```python
from build123d import *

# Parameters (mm, degrees)
F0_W      = 76.2
F0_H      = 44.45
F1_DEPTH  = 25.4
F2_W      = 25.4
F2_H      = 31.75
F3_DEPTH  = 25.4
F5_DEPTH  = 25.4
F6_R      = 6.4097616639
F7_DEPTH  = 25.4
F9_DEPTH  = 25.4
F11_DEPTH = 25.4
F12_R     = 6.9616762065
F12_R_2   = 6.701591824
F13_DEPTH = 25.4


with BuildPart() as f1:
    # F0 (on Front) → F1 (new body)
    with BuildSketch(Plane.XZ):
        with Locations((38.1, 22.225)):
            Rectangle(F0_W, F0_H)
    extrude(amount=F1_DEPTH)

    # F2 (on face) → F3 (cut)
    with BuildSketch(Plane.XZ.offset(25.4)):
        with Locations((12.7, 28.575)):
            Rectangle(F2_W, F2_H)
        with Locations((63.5, 28.575)):
            Rectangle(F2_W, F2_H)
    extrude(amount=-F3_DEPTH, mode=Mode.SUBTRACT)

    # F4 (on face) → F5 (cut)
    with BuildSketch(Plane.YZ.offset(50.8)):
        with BuildLine():
            ThreePointArc((-25.4, 37.343819084), (-21.8851025395, 42.054991557), (-16.517273855, 44.45))
            Line((-16.517273855, 44.45), (-25.4, 44.45))
            Line((-25.4, 44.45), (-25.4, 37.343819084))
        make_face()
        with BuildLine():
            Line((0, 44.45), (-12.7, 44.45))
            ThreePointArc((-12.7, 44.45), (-4.2917980427, 40.8099765707), (0, 32.7150336876))
            Line((0, 32.7150336876), (0, 44.45))
        make_face()
    extrude(amount=-F5_DEPTH, mode=Mode.SUBTRACT)

    # F6 (on face) → F7 (cut)
    with BuildSketch(Plane.YZ.offset(50.8)):
        with Locations((-13.6843539452, 30.6450168438)):
            Circle(F6_R)
    extrude(amount=-F7_DEPTH, mode=Mode.SUBTRACT)

    # F8 (on face) → F9 (cut)
    with BuildSketch(Plane.XY.offset(12.7)):
        with BuildLine():
            Line((0, 0), (0, -9.0078908736))
            ThreePointArc((0, -9.0078908736), (2.3832082238, -3.5743776274), (7.1188784204, 0))
            Line((7.1188784204, 0), (0, 0))
        make_face()
        with BuildLine():
            ThreePointArc((7.1188784204, -25.4), (2.2814327848, -21.4359106329), (0, -15.612685647))
            Line((0, -15.612685647), (0, -25.4))
            Line((0, -25.4), (7.1188784204, -25.4))
        make_face()
    extrude(amount=-F9_DEPTH, mode=Mode.SUBTRACT)

    # F10 (on face) → F11 (cut)
    with BuildSketch(Plane.XY.offset(12.7)):
        with BuildLine():
            ThreePointArc((67.3354417086, 0), (73.7069873412, -4.7726544119), (76.2, -12.3330586186))
            Line((76.2, -12.3330586186), (76.2, 0))
            Line((76.2, 0), (67.3354417086, 0))
        make_face()
        with BuildLine():
            ThreePointArc((76.2, -14.8152652197), (73.4320785831, -21.5015075072), (67.3354417086, -25.4))
            Line((67.3354417086, -25.4), (76.2, -25.4))
            Line((76.2, -25.4), (76.2, -14.8152652197))
        make_face()
    extrude(amount=-F11_DEPTH, mode=Mode.SUBTRACT)

    # F12 (on face) → F13 (cut)
    with BuildSketch(Plane.XY.offset(12.7)):
        with Locations((62.8318414092, -12.3102882603)):
            Circle(F12_R)
        with Locations((15.475823544, -12.3102882603)):
            Circle(F12_R_2)
    extrude(amount=-F13_DEPTH, mode=Mode.SUBTRACT)


solid = f1.part
```
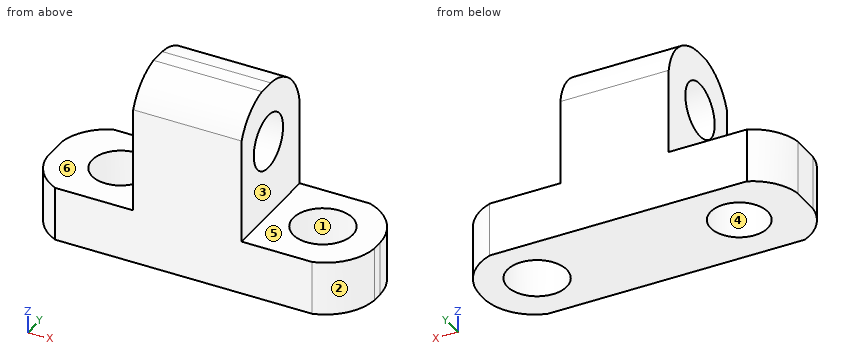
Input: part model. Units: mm. Frame: model coordinates. Face numbers are marked on the shaded views. A direction names the side the tool comes from. Round coordinates to 2 decimals unless told otherwise and drop trailing zeros. Order: outer loops, then holes, each group sorted by start corner. A loop starts at its lowest first (then second) coordinate and runs counter-clockwise, first axis right, second up. Notation, with made-up numbers: (61.25, 80) - (65.25, 80) arc R27 ccw to (65.25, 112) - close; hole circle Ø3 at (-39.75, 69). An arc over 180 degrees is marked (long way). Answer in a Markdown table with one row per item.
Item 1: Section query D-D (x = 42.5). Return the cut outline in (y, z).
Model answer:
| item | result |
|---|---|
| outline | (-25.4, 0) - (0, 0) - (0, 32.72) arc R13.84 ccw to (-12.7, 44.45) - (-16.52, 44.45) arc R11.65 ccw to (-25.4, 37.34) - close; hole circle Ø12.82 at (-13.68, 30.65) |
Item 2: Reachability of the marked faces 4, 5 and 6 from +Z, -Z, +X, -X, +Y, -Y: full face, straight path, thin tool, end or side. Return the list, or none.
Model answer:
| item | result |
|---|---|
| face 4 | +Z, -Z |
| face 5 | +Z, +X, +Y, -Y |
| face 6 | +Z, -X, +Y, -Y |
Item 3: Pin query (flat end, axial travel): pin 1 (10.5 mm diameter, centred on y = -13.68, z = 30.65, fed in from +X); pin 2 (1.5 mm diameter, centred on y = -17, z = 15.5, fed in from -X); pin 3 (8 mm diameter, centred on y = -17, z = 22.5, fed in from +X); pin 4 (7.5 mm diameter, centred on x = 15.5, y = -6.5, fed in from +Z). Return the tip coordinate at first contact, or that it passes through.
Model answer:
| item | result |
|---|---|
| pin 1 | passes through |
| pin 2 | stops at x = 25.4 |
| pin 3 | stops at x = 50.8 |
| pin 4 | stops at z = 12.7 |
Item 4: Section query C-C (z = 7.5). Return the cut outline in (x, y).
Model answer:
| item | result |
|---|---|
| outline | (0, -15.61) arc R12.38 ccw to (7.12, -25.4) - (67.34, -25.4) arc R12.06 ccw to (76.2, -14.82) - (76.2, -12.33) arc R13.27 ccw to (67.34, 0) - (7.12, 0) arc R11.74 ccw to (0, -9.01) - close; hole circle Ø13.4 at (15.48, -12.31); hole circle Ø13.92 at (62.83, -12.31) |
Item 5: Line query: line 1 (X direction, y = -12, z = 5); line 2 (X direction, y = -13, z = 38.5); line 3 (Z direction, x = 55, y = -10.5). Output: solid intervals per line, ascending.
Model answer:
| item | result |
|---|---|
| line 1 | x = 0 to 8.78, 22.17 to 55.88, 69.79 to 76.19 |
| line 2 | x = 25.4 to 50.8 |
| line 3 | z = 0 to 12.7 |
Item 6: Section query A-A (x = 59). Return the cut outline in (y, z).
Model answer:
| item | result |
|---|---|
| outline | (-25.4, 0) - (-18.12, 0) - (-18.12, 12.7) - (-25.4, 12.7) - close; (-6.5, 0) - (0, 0) - (0, 12.7) - (-6.5, 12.7) - close |
Item 7: Mould query, pull axis Y, two halves, no side actions, for the marked faces 1, 2 and 3. Classes: released by +Y, released by -Y, zero draft, split by the parting line, or undercut.
Model answer:
| item | result |
|---|---|
| face 1 | undercut |
| face 2 | released by -Y |
| face 3 | zero draft |
Item 8: Section query B-B (z = 25). Return the cut outline in (x, y), then the cut area to 3 significant figures.
Model answer:
| item | result |
|---|---|
| outline | (25.4, -25.4) - (50.8, -25.4) - (50.8, -16.72) - (25.4, -16.72) - close; (25.4, -10.65) - (50.8, -10.65) - (50.8, 0) - (25.4, 0) - close |
| area | 491 mm² |
